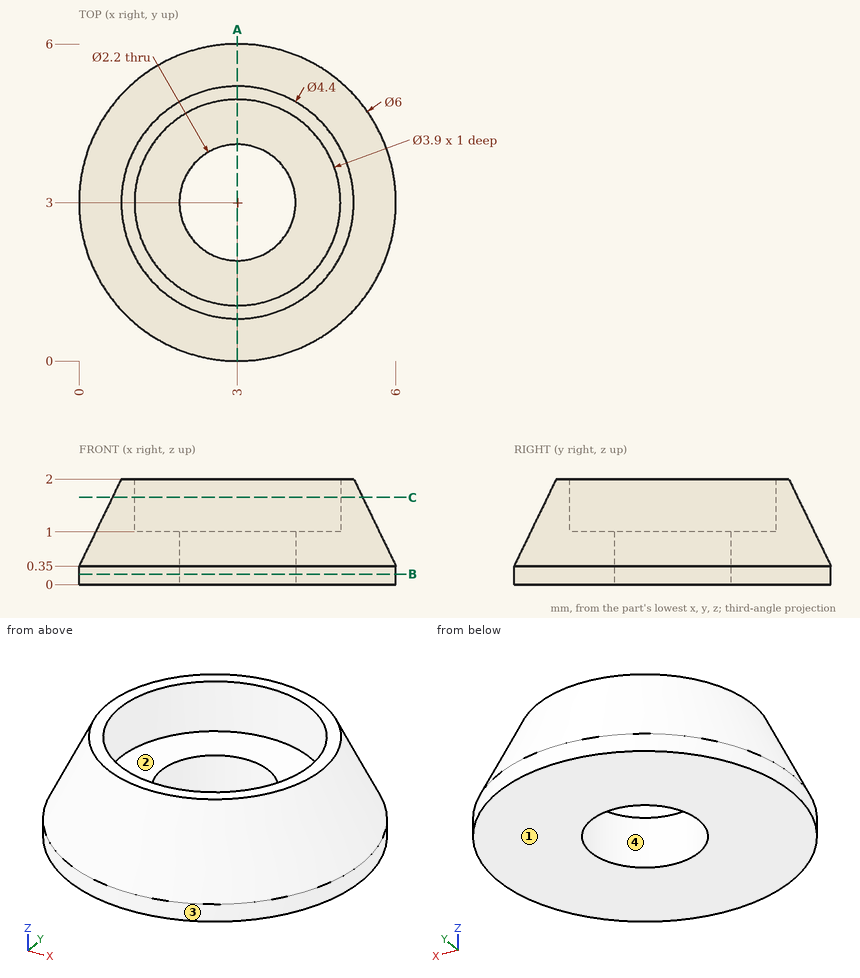
Check sheet for the drawn part. Datum: minimum x, y, z corner. Units: mm. Round coordinates to 2 decimals unless told otherwise and drop trailing zeros. Order: outer loops, then holes, each group sorted by start corner. A loop starts at its lowest first (then second) coordinate and runs counter-clockwise, first axis right, second up. Notation, with made-up numbers: (-31, 74.25) -> (0, 74.25) arc R22 ccw to (0, 94.25) -> close; hole circle Ø5 at (55.25, 1). An arc over 180 degrees is marked (long way). Put each result on its own line as item: value.
1) Mould release check, pull along Y, two halves, no side actions. Record for the marked faces 1, 2, 3 and 4: +Y half, -Y half, draft (parallel to the pull), parting line (faces both ways), or undercut.
Final values:
face 1: draft
face 2: undercut
face 3: parting line
face 4: undercut
2) Section check B-B (z = 0.2). Record the cut outline in (x, y), then the cut area to 3 significant figures.
Final values:
outline: circle Ø6 at (3, 3); hole circle Ø2.2 at (3, 3)
area: 24.5 mm^2
3) Material ranges on line 1 (Y direction, x = 4, z = 1.8); line 2 (Z direction, x = 1.75, y = 4.25); line 3 (Y direction, x = 3, z = 1.4), recorded low to high.
Final values:
line 1: y = 0.93 to 1.33, 4.67 to 5.07
line 2: z = 0 to 1
line 3: y = 0.51 to 1.05, 4.95 to 5.49
4) Depth check by flat-ended pin: pin 1 (3 mm diameter, centred on x = 1.5, y = 3, fed in from +Z); pin 2 (3 mm diameter, centred on x = 3, y = 3, fed in from +Z). Enter the tip coordinate at first touch or a pass-through.
Final values:
pin 1: stops at z = 2
pin 2: stops at z = 1
5) Section check C-C (z = 1.65). Record the cut outline in (x, y).
Final values:
outline: circle Ø4.74 at (3, 3); hole circle Ø3.9 at (3, 3)
6) Section check A-A (x = 3). Record the cut outline in (y, z), then the cut area to 3 significant figures.
Final values:
outline: (0, 0) -> (1.9, 0) -> (1.9, 1) -> (1.05, 1) -> (1.05, 2) -> (0.8, 2) -> (0, 0.35) -> close; (4.1, 0) -> (6, 0) -> (6, 0.35) -> (5.2, 2) -> (4.95, 2) -> (4.95, 1) -> (4.1, 1) -> close
area: 4.58 mm^2
